Autodesk Inventor part; units mm, degrees
ref_plane "YZ Plane" through (0, 0, 0) normal (1, 0, 0) x (0, 1, 0)
ref_plane "XZ Plane" through (0, 0, 0) normal (0, 1, 0) x (-1, 0, 0)
ref_plane "XY Plane" through (0, 0, 0) normal (0, 0, 1) x (1, 0, 0)
sketch "草图1" plane through (0, 0, 0) normal (0, 1, 0) x (-1, 0, 0)
  line L0 (0, 0) -> (68, 0)
  line L1 (68, 0) -> (68, -280)
  line L2 (68, -280) -> (0, -280)
  line L3 (0, -280) -> (0, 0)
  line L4 (34, 0) -> (34, -21)
  circle A0 centre (34, -21) radius 2
  line L5 (34, -21) -> (34, -46)
  circle A1 centre (34, -46) radius 2
  line L6 (34, -46) -> (34, -101)
  line L7 (34, -101) -> (44, -101)
  line L8 (34, -101) -> (24, -101)
  circle A2 centre (44, -101) radius 1.5
  circle A3 centre (24, -101) radius 1.5
  line L9 (34, -101) -> (34, -166)
  line L10 (34, -166) -> (44, -166)
  line L11 (34, -166) -> (24, -166)
  circle A4 centre (44, -166) radius 1.5
  circle A5 centre (24, -166) radius 1.5
  line L12 (34, -166) -> (34, -232)
  line L13 (34, -232) -> (44, -232)
  line L14 (34, -232) -> (24, -232)
  circle A6 centre (44, -232) radius 1.5
  circle A7 centre (24, -232) radius 1.5
  dimension "d0" = 68
  dimension "d1" = 280
  dimension "d2" = 21
  dimension "d3" = 4
  dimension "d4" = 25
  dimension "d5" = 4
  dimension "d6" = 55
  dimension "d7" = 10
  dimension "d8" = 10
  dimension "d9" = 3
  dimension "d10" = 3
  dimension "d11" = 65
  dimension "d12" = 10
  dimension "d13" = 10
  dimension "d14" = 3
  dimension "d15" = 3
  dimension "d16" = 66
  dimension "d17" = 10
  dimension "d18" = 10
  dimension "d19" = 3
  dimension "d20" = 3
extrude "拉伸1" add sketch "草图1" along normal blind 3
sketch "草图3" plane through (0, 0, 0) normal (0, -1, 0) x (1, 0, 0)
  line L0 (0, -280) -> (-68, -280)
  line L1 (-68, 0) -> (0, 0)
  line L2 (-68, -280) -> (-66, -280)
  line L3 (-66, -280) -> (-66, 0)
  line L4 (-66, 0) -> (-68, 0)
  line L5 (-68, 0) -> (-68, -280)
  dimension "d26" = 2
extrude "拉伸3" add sketch "草图3" along normal blind 200
equation "\"折弯半径\" = 厚度"
equation "\"折弯释压宽度\" = 厚度"
equation "\"折弯释压深度\" = 0.5 * 厚度"
equation "\"拐角释压尺寸\" = 4 * 厚度"
equation "\"最小余量\" = 2 * 厚度"
equation "\"过渡半径\" = 折弯半径"
equation "\"Jacobi半径尺寸\" = 折弯半径"
equation "\"间隙大小\" = 厚度"
properties part number "底板3"
Part model, mm, in its own coordinate system. A direction names the side the tool comes from. Give positions to 0.01 mm unless a question says otherwise; leave off trailing zeros. Write each loop counter-clockwise with the first axis right and the second up, starting at its lowest first coordinate (ties: lowest second). Pieces come first, ordered by that corner, then holes. Notation, with made-up numbers: (62, -19.75) -> (121, -19.75) arc R13 ccw to (121, 5.25) -> close; hole circle Ø5 at (15.25, 77.25). An arc over 180 degrees is marked (long way). Put each result on its own line as item: value. Start each with the question number.
Item 1: Pin check, flat tips, straight feed: pin 1 Ø5 at (x, z) = (-24, -232) entering from -Y; pin 2 Ø4 at (y, z) = (-80, -195.5) entering from +X. Stop position of each tip, or through.
Item 2: Which spindle directions (+Z, -Z, +X, -X, +Y, -Y) get a long thin tool onto all of the face, cutting with end or side? Do faces 1 (the face through (-66, -99, -142)), 2 (the face through (-67, -99, -280)). Say none if no direction does.
Item 3: Cut at C-C (y = -63). List the corners of the cut face in (x, z), then the cut area to 3 significant figures.
Item 4: Wall check: L1, parallel to X at y = 1, z = -232; L2, parallel to Z at x = -44, y = 1.45; L3, parallel to Z at x = -34, y = 1.2. Give the ranges that are in metal, low to high. Write a range as [from, to].
Item 5: Cut at A-A (z = -41). List the corners of the cut face in (x, y), then the cut area to 3 significant figures.
Item 6: Cut at B-B (x = -62.5). List the corners of the cut face in (y, z).
Answer list:
1. pin 1: stops at y = 0
1. pin 2: stops at x = -66
2. face 1: +Z, -Z, +X, -Y
2. face 2: -Z, +X, -X, +Y, -Y
3. outline: (-68, -280) -> (-66, -280) -> (-66, 0) -> (-68, 0) -> close
3. area: 560 mm2
4. L1: x = [-68, -45.5], [-42.5, -25.5], [-22.5, 0]
4. L2: z = [-280, -233.5], [-230.5, -167.5], [-164.5, -102.5], [-99.5, 0]
4. L3: z = [-280, -48], [-44, -23], [-19, 0]
5. outline: (-68, -200) -> (-66, -200) -> (-66, 0) -> (0, 0) -> (0, 3) -> (-68, 3) -> close
5. area: 604 mm2
6. outline: (0, -280) -> (3, -280) -> (3, 0) -> (0, 0) -> close
